The listing builds one solid part. Answer for the finished solid, in the listing's coordinates (mm). A direction names the side the tool comes from. Round coordinates to 2 decimals unless told otherwise and drop trailing zeros. Write each loop counter-clockwise with the first axis right and the second up, starting at its lowest first coordinate (ties: lowest second). Pieces come first, ordered by that corner, then holes. Notation, with made-up numbers: (23, 12.5) - (63, 12.5) arc R22 ccw to (63, 46.5) - close; hole circle Ø7 at (81.25, -25). An arc over 180 degrees is marked (long way). Use a Markdown table: item, result. Add a question column.
1) A cutting plane is placed at C-C (y = 161). Give the vertices of the cut face in (x, z), then the cut area to 4 significant figures.
2) Determine the mould class of faces 6 (the cylindrical face through (-211.997, -1.164, 9.86)), 7 (the flat face through (-78, 187, 12)), 8 (the flat face through (-63.5, -68, 10)) for opening direction X: +X half, -X half, draft (parallel to the pull), parting line (faces both ways), or undercut.
3) A cutting plane is placed at A-A (x = -158). Give the vertices of the cut face in (y, z).
4) A cutting plane is placed at D-D (x = -87). Give the vertices of the cut face in (y, z), then the cut area to 3 significant figures.
5) A cutting plane is placed at B-B (z = 12). Give the vertices of the cut face in (x, y), then the cut area to 3 significant figures.
6) Find the intervals of material crossed by probe 1 along Y at (x, z) = (-138.5, 12.5); probe 2 along Y at (x, z) = (-99.5, 1.5); probe 3 along X at (y, z) = (100.5, 3.75), in increasing order. Write a range as from..to.
7) A tool of negligible diameter and unlimited length cuts with its end or side. For faces 1 (the flat face through (-78, 190, 10)), 2 (the flat face through (-144, 81, 10)), 3 (the flat face through (-119, -56, 10)), 4 (the cylindrical face through (-70.19, 82.91, 10.14)), 5 (the flat face through (-66.5, -69, 12)), from which of +Z, -Z, +X, -X, +Y, -Y can it reach the whole face along a straight path? Write none if from no direction.
8) Each of these flat-tipped pins is pushed along its axis until it touches: P1, Ø10, axis at x = -136, z = 7.5, coming from the +Y side; P2, Ø8.5, axis at y = 124.5, z = 14, coming from the +X side; P3, Ø4, axis at y = 55.5, z = 13.5, coming from the -X side. Where does it stop, or does it pass through?
```python
from build123d import *

# Parameters (mm, degrees)
BOSS_EXTRUDE1_DEPTH = 20
CUT_EXTRUDE1_DEPTH  = 17
FILLET1_R           = 6.35


with BuildPart() as part:
    # Sketch1 → Boss-Extrude1 (new body)
    with BuildSketch(Plane.XY):
        with BuildLine():
            Line((-195.91579824, 81), (-84.5, 81))
            Line((-84.5, 81), (-84.5, 190))
            Line((-84.5, 190), (-72, 190))
            Line((-72, 190), (-72, 81))
            Line((-72, 81), (-63.5, 81))
            Line((-63.5, 81), (-63.5, 56))
            Line((-63.5, 56), (-178.418048414, 56))
            ThreePointArc((-178.418048414, 56), (-187, 0), (-178.418048414, -56))
            Line((-178.418048414, -56), (-63.5, -56))
            Line((-63.5, -56), (-63.5, -81))
            Line((-63.5, -81), (-195.91579824, -81))
            ThreePointArc((-195.91579824, -81), (-212, 0), (-195.91579824, 81))
        make_face()
    extrude(amount=BOSS_EXTRUDE1_DEPTH)

    # Sketch2 → Cut-Extrude1 (cut)
    with BuildSketch(Plane.XY.offset(20)):
        with BuildLine():
            Line((-66.5, 78), (-75, 78))
            Line((-75, 78), (-75, 187))
            Line((-75, 187), (-81.5, 187))
            Line((-81.5, 187), (-81.5, 78))
            Line((-81.5, 78), (-193.899458483, 78))
            ThreePointArc((-193.899458483, 78), (-209, 0), (-193.899458483, -78))
            Line((-193.899458483, -78), (-66.5, -78))
            Line((-66.5, -78), (-66.5, -59))
            Line((-66.5, -59), (-180.607308822, -59))
            ThreePointArc((-180.607308822, -59), (-190, 0), (-180.607308822, 59))
            Line((-180.607308822, 59), (-66.5, 59))
            Line((-66.5, 59), (-66.5, 78))
        make_face()
    extrude(amount=-CUT_EXTRUDE1_DEPTH, mode=Mode.SUBTRACT)

    # Fillet1
    fillet1_edges = [part.edges().sort_by_distance(p)[0] for p in [
        (-178.418048414, 56, 10),
        (-178.418048414, -56, 10),
        (-84.5, 81, 10),
        (-72, 81, 10),
    ]]
    fillet(fillet1_edges, radius=FILLET1_R)


solid = part.part
```
Entries:
| question | item | result |
|---|---|---|
| 1 | outline | (-84.5, 0) - (-72, 0) - (-72, 20) - (-75, 20) - (-75, 3) - (-81.5, 3) - (-81.5, 20) - (-84.5, 20) - close |
| 1 | area | 139.5 mm² |
| 2 | face 6 | -X half |
| 2 | face 7 | undercut |
| 2 | face 8 | +X half |
| 3 | outline | (-81, 0) - (-56, 0) - (-56, 20) - (-59, 20) - (-59, 3) - (-78, 3) - (-78, 20) - (-81, 20) - close; (56, 0) - (81, 0) - (81, 20) - (78, 20) - (78, 3) - (59, 3) - (59, 20) - (56, 20) - close |
| 4 | outline | (-81, 0) - (-56, 0) - (-56, 20) - (-59, 20) - (-59, 3) - (-78, 3) - (-78, 20) - (-81, 20) - close; (56, 0) - (82.3, 0) - (82.3, 20) - (78, 20) - (78, 3) - (59, 3) - (59, 20) - (56, 20) - close |
| 4 | area | 380 mm² |
| 5 | outline | (-195.92, -81) - (-63.5, -81) - (-63.5, -56) - (-173.69, -56) arc R6.35 cw to (-179.8, -51.4) arc R187 cw to (-179.8, 51.4) arc R6.35 cw to (-173.69, 56) - (-63.5, 56) - (-63.5, 81) - (-65.65, 81) arc R6.35 cw to (-72, 87.35) - (-72, 190) - (-84.5, 190) - (-84.5, 87.35) arc R6.35 cw to (-90.85, 81) - (-195.92, 81) arc R212 ccw to start; hole (-193.9, -78) - (-66.5, -78) - (-66.5, -59) - (-180.61, -59) arc R190 cw to (-180.61, 59) - (-66.5, 59) - (-66.5, 78) - (-75, 78) - (-75, 187) - (-81.5, 187) - (-81.5, 78) - (-193.9, 78) arc R209 ccw to start |
| 5 | area | 3,120 mm² |
| 6 | probe 1 | y = -81..-78, -59..-56, 56..59, 78..81 |
| 6 | probe 2 | y = -81..-56, 56..81 |
| 6 | probe 3 | x = -84.5..-81.5, -75..-72 |
| 7 | face 1 | +Z, -Z, +X, -X, +Y |
| 7 | face 2 | +Z, -Z, -X, +Y |
| 7 | face 3 | +Z, -Z, +X |
| 7 | face 4 | +Z, -Z, +X, +Y |
| 7 | face 5 | +Z |
| 8 | P1 | stops at y = 81 |
| 8 | P2 | stops at x = -72 |
| 8 | P3 | stops at x = -205.14 |
